```python
from build123d import *

# Parameters (mm, degrees)
SKETCH_1_W      = 58
SKETCH_1_H      = 20
SKETCH_1_R      = 1.75
EXTRUDE_1_DEPTH = 38
FILLET_1_R      = 5


with BuildPart() as part:
    # 草图1 → 凸台-拉伸1 (new body)
    with BuildSketch(Plane.XY):
        Rectangle(SKETCH_1_W, SKETCH_1_H)
        with Locations((-20, 6)):
            Circle(SKETCH_1_R, mode=Mode.SUBTRACT)
        with Locations((-8, 6)):
            Circle(SKETCH_1_R, mode=Mode.SUBTRACT)
        with Locations(Location((8, 6, 0), (0, 0, 180))):
            Circle(SKETCH_1_R, mode=Mode.SUBTRACT)
        with Locations(Location((20, 6, 0), (0, 0, 180))):
            Circle(SKETCH_1_R, mode=Mode.SUBTRACT)
        with Locations((-20, -4)):
            Circle(SKETCH_1_R, mode=Mode.SUBTRACT)
        with Locations((-8, -4)):
            Circle(SKETCH_1_R, mode=Mode.SUBTRACT)
        with Locations(Location((8, -4, 0), (0, 0, 180))):
            Circle(SKETCH_1_R, mode=Mode.SUBTRACT)
        with Locations(Location((20, -4, 0), (0, 0, 180))):
            Circle(SKETCH_1_R, mode=Mode.SUBTRACT)
    extrude(amount=EXTRUDE_1_DEPTH)

    # 圆角1
    fillet_1_edges = [part.edges().sort_by_distance(p)[0] for p in [
        (-29, 0, 38),
        (29, 0, 38),
        (-29, 0, 0),
        (29, 0, 0),
    ]]
    fillet(fillet_1_edges, radius=FILLET_1_R)


solid = part.part
```
Source: CAD feature listing. Evaluate the final solid. Frame: model axes, mm. Give positions to 0.01 mm unless a question says otherwise; leave off trailing zeros. Loops run counter-clockwise (first coordinate to the right, second up) from the corner with the lowest first, then second, coordinate; pieces in that order, holes last. Notation, with made-up numbers: (86, 42.25) -> (93, 42.25) arc R15 cw to (93, 57.25) -> close; hole circle Ø4 at (24, -24). An arc over 180 degrees is marked (long way). Put each result on its own line as item: value. Start each with the question number.
1) Material intervals for probe 1 along Y at (x, z) = (8, 10); probe 2 along X at (y, z) = (5.5, 34.5); probe 3 along X at (y, z) = (-4.5, 11.5), sorted ascending.
2) Cut plane D-D (y = 5). Return loops of the section in (x, z).
3) Cut plane C-C (z = 17). State how many separate pieces and enclosed holes the cut face has, then the cut area to 3 significant figures.
4) Contact query for a flat-ended pin moving along its axis: P1, Ø3, axis at x = -8, y = -4, coming from the +Z side. Output: stop coordinate, or through.
5) Draft query along Y for faces 1 (the face through (6.383, -3.33, 18.734)), 2 (the face through (29, 0, 19)), 3 (the face through (21.75, -4.08, 18.73)), 4 (the face through (0, -10, 19)). Return one class per face: released by +Y, released by -Y, zero draft, split by the parting line, or undercut.
6) Cut plane A-A (y = -4). Return loops of the section in (x, z), then the cut area to 3 significant figures.
7) Cut plane B-B (x = -8). Return loops of the section in (y, z).
Results are:
1. probe 1: y = -10 to -5.75, -2.25 to 4.25, 7.75 to 10
1. probe 2: x = -28.77 to -21.68, -18.32 to -9.68, -6.32 to 6.32, 9.68 to 18.32, 21.68 to 28.77
1. probe 3: x = -29 to -21.68, -18.32 to -9.68, -6.32 to 6.32, 9.68 to 18.32, 21.68 to 29
2. outline: (-29, 5) arc R5 ccw to (-24, 0) -> (-21.44, 0) -> (-21.44, 38) -> (-24, 38) arc R5 ccw to (-29, 33) -> close; (-18.56, 0) -> (-9.44, 0) -> (-9.44, 38) -> (-18.56, 38) -> close; (-6.56, 0) -> (6.56, 0) -> (6.56, 38) -> (-6.56, 38) -> close; (9.44, 0) -> (18.56, 0) -> (18.56, 38) -> (9.44, 38) -> close; (21.44, 0) -> (24, 0) arc R5 ccw to (29, 5) -> (29, 33) arc R5 ccw to (24, 38) -> (21.44, 38) -> close
3. separate pieces: 1
3. enclosed holes: 8
3. area: 1,080 mm2
4. P1: passes through
5. face 1: undercut
5. face 2: zero draft
5. face 3: undercut
5. face 4: released by -Y
6. outline: (-29, 5) arc R5 ccw to (-24, 0) -> (-21.75, 0) -> (-21.75, 38) -> (-24, 38) arc R5 ccw to (-29, 33) -> close; (-18.25, 0) -> (-9.75, 0) -> (-9.75, 38) -> (-18.25, 38) -> close; (-6.25, 0) -> (6.25, 0) -> (6.25, 38) -> (-6.25, 38) -> close; (9.75, 0) -> (18.25, 0) -> (18.25, 38) -> (9.75, 38) -> close; (21.75, 0) -> (24, 0) arc R5 ccw to (29, 5) -> (29, 33) arc R5 ccw to (24, 38) -> (21.75, 38) -> close
6. area: 1,650 mm2
7. outline: (-10, 0) -> (-5.75, 0) -> (-5.75, 38) -> (-10, 38) -> close; (-2.25, 0) -> (4.25, 0) -> (4.25, 38) -> (-2.25, 38) -> close; (7.75, 0) -> (10, 0) -> (10, 38) -> (7.75, 38) -> close
